Can you work these out from the model? Positions are in its coordinate system, mm. Face numbers are marked on the shaded views. A direction names the side the tool comes from. Give positions to 0.01 mm unless a question says otherwise; leave off trailing zeros. Loops run counter-clockwise (first coordinate to the right, second up) from the corner with the lowest first, then second, coordinate; pieces in that order, holes last. Notation, with made-up numbers: M 5,-6.75 L 56,-6.75 A18 ccw 56,11.25 Z; hole C 58,52.5 d2. An arc over 180 degrees is marked long. One line per item, written item: value. Start each with the question number.
from build123d import *

# Parameters (mm, degrees)
SKETCH_1_W          = 27
SKETCH_1_H          = 10
EXTRUDE_1_DEPTH     = 34.7
SKETCH_2_W          = 12
SKETCH_2_H          = 5
CUT_EXTRUDE_1_DEPTH = 35.7
HOLE_WIZARD_M3_1_D  = 2.5


with BuildPart() as part:
    # 草图1 → 凸台-拉伸1 (new body)
    with BuildSketch(Plane.XY):
        with Locations((13.5, 5)):
            Rectangle(SKETCH_1_W, SKETCH_1_H)
    extrude(amount=EXTRUDE_1_DEPTH)

    # 草图2 → 切除-拉伸1 (cut, through all)
    with BuildSketch(Plane(origin=(0, 0, 0), x_dir=(-1, 0, 0), z_dir=(0, 0, -1))):
        with Locations((-13.5, 2.5)):
            Rectangle(SKETCH_2_W, SKETCH_2_H)
    extrude(amount=-CUT_EXTRUDE_1_DEPTH, mode=Mode.SUBTRACT)

    # M3 螺纹孔1 (through all)
    with Locations(Plane(origin=(0, 10, 0), x_dir=(1, 0, 0), z_dir=(0, 1, 0))):
        with Locations((23.5, -24.85), (23.5, -9.85), (3.5, -24.85), (3.5, -9.85)):
            Hole(HOLE_WIZARD_M3_1_D / 2)


solid = part.part
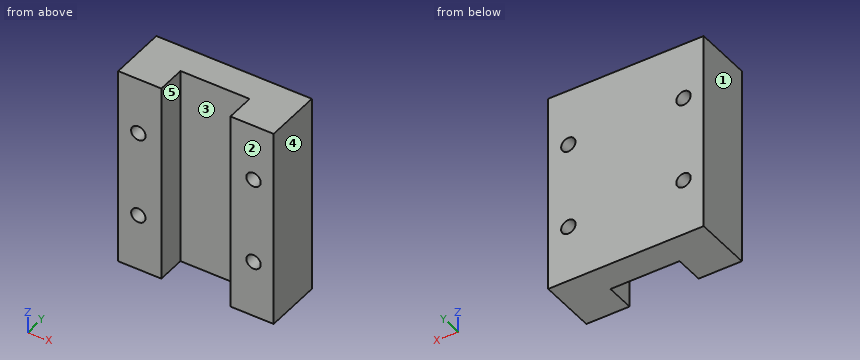
Q1. For P1, Ø3, axis at x = 23.5, z = 9.85, coming from the -Y side; P2, Ø3.5, axis at x = 14, z = 21, coming from the -Y side; P3, Ø1.5, axis at x = 23.5, z = 24.85, coming from the +Y side, each with a flat end and sliding along its axis, tell me the tip position at first contact or that it passes through.
Q2. Which directions (+Z, -Z, +X, -X, +Y, -Y) give clear straight access to the entire face, cutting with the end or side of a thin tool? Please do the marked faces 4 and 5.
Q3. If we section it at B-B, the plane z = 24.85: Write out the boundary of the cut face in (x, y).
Q4. If we section it at D-D, the plane z = 29.5: Write out the boundary of the cut face in (x, y).
Q5. If we mould it in two halves opening along X, with no side actions, what happens to the marked faces 1, 2 and 3? For each: released by +X, released by -X, zero draft, split by the parting line, or undercut.
Q6. If we section it at A-A, the plane y = 2: Write out the boundary of the cut face in (x, z).
Q7. I need wall thicknesses on line 1 along Z through (x, y) = (23.5, 5.75); line 2 along X through (y, z) = (4, 9.85); line 3 along X through (y, z) = (2.25, 31.5). Which ranges of each line are inside material? Lowest first, please.
Q8. If we section it at C-C, the plane x = 3.5: Write out the boundary of the cut face in (y, z), plus the area to 3 significant figures.
Response:
1. P1: y = 0
1. P2: y = 5
1. P3: through
2. face 4: +Z, -Z, +X, +Y, -Y
2. face 5: +Z, -Z, -Y
3. outline: M 0,0 L 2.25,0 L 2.25,10 L 0,10 Z; M 4.75,0 L 7.5,0 L 7.5,5 L 19.5,5 L 19.5,0 L 22.25,0 L 22.25,10 L 4.75,10 Z; M 24.75,0 L 27,0 L 27,10 L 24.75,10 Z
4. outline: M 0,0 L 7.5,0 L 7.5,5 L 19.5,5 L 19.5,0 L 27,0 L 27,10 L 0,10 Z
5. face 1: released by -X
5. face 2: zero draft
5. face 3: undercut
6. outline: M 0,0 L 7.5,0 L 7.5,34.7 L 0,34.7 Z; M 19.5,0 L 27,0 L 27,34.7 L 19.5,34.7 Z; hole C 3.5,9.85 d2.5; hole C 3.5,24.85 d2.5; hole C 23.5,9.85 d2.5; hole C 23.5,24.85 d2.5
7. line 1: 0 to 8.6, 11.1 to 23.6, 26.1 to 34.7
7. line 2: 0 to 2.25, 4.75 to 7.5, 19.5 to 22.25, 24.75 to 27
7. line 3: 0 to 7.5, 19.5 to 27
8. outline: M 0,0 L 10,0 L 10,8.6 L 0,8.6 Z; M 0,11.1 L 10,11.1 L 10,23.6 L 0,23.6 Z; M 0,26.1 L 10,26.1 L 10,34.7 L 0,34.7 Z
8. area: 297 mm^2
